from build123d import *

# Parameters (mm, degrees)
SKETCH1_W           = 11
SKETCH1_H           = 12
BOSS_EXTRUDE1_DEPTH = 6.6
CUT_EXTRUDE1_DEPTH  = 6.6


with BuildPart() as part:
    # Sketch1 → Boss-Extrude1 (new body)
    with BuildSketch(Plane(origin=(0, 0, 0), x_dir=(1, 0, 0), z_dir=(0, 1, 0))):
        with Locations((5.5, -6)):
            Rectangle(SKETCH1_W, SKETCH1_H)
    extrude(amount=BOSS_EXTRUDE1_DEPTH)

    # Sketch2 → Cut-Extrude1 (cut)
    with BuildSketch(Plane(origin=(0, 6.6, 0), x_dir=(1, 0, 0), z_dir=(0, 1, 0))):
        with BuildLine():
            ThreePointArc((11, -0.013348181), (9.4, -6), (11, -11.986651819))
            Line((11, -11.986651819), (11, -0.013348181))
        make_face()
        with BuildLine():
            ThreePointArc((0, -11.986651819), (1.6, -6), (0, -0.013348181))
            Line((0, -0.013348181), (0, -11.986651819))
        make_face()
        with BuildLine():
            ThreePointArc((7.275, -6), (6.755114537, -4.744885463), (5.5, -4.225))
            Line((5.5, -4.225), (5.5, -7.775))
            ThreePointArc((5.5, -7.775), (6.755114537, -7.255114537), (7.275, -6))
        make_face()
        with BuildLine():
            Line((5.5, -7.775), (5.5, -4.225))
            ThreePointArc((5.5, -4.225), (3.725, -6), (5.5, -7.775))
        make_face()
    extrude(amount=-CUT_EXTRUDE1_DEPTH, mode=Mode.SUBTRACT)


solid = part.part
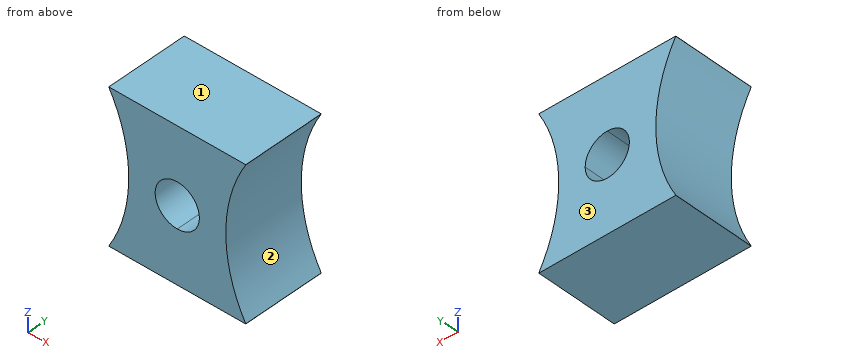
For this review, take the finished solid that the model builds, in its own axes (mm). Face numbers are marked on the shaded views. Round coordinates to 2 decimals unless told otherwise and drop trailing zeros. Loops run counter-clockwise (first coordinate to the right, second up) from the corner with the lowest first, then second, coordinate; pieces in that order, holes last. Notation, with made-up numbers: (40.5, 58) - (48.5, 58) arc R23 ccw to (48.5, 89) - close; hole circle Ø11 at (17, -17.75). An arc over 180 degrees is marked (long way). Put each result on its own line as item: value. Start each with the question number.
1. For probe 1 along Z at (x, y) = (4.5, 2); probe 2 along X at (y, z) = (2.75, 5.25); probe 3 along Z at (x, y) = (6.25, 0.5), list the stretches that pass through material, from the lowest coordinate up. Write a range as [from, to].
2. Consider section A-A on y = 3.75. State the section outline as (x, z) points (3 decimals).
3. Mouldability with a two-part tool opening along Z and no side actions: class the marked faces 1, 2 and 3 as +Z half, -Z half, draft (parallel to the pull), parting line (faces both ways), or undercut.
4. Insertion check: P1, Ø1.5, axis at x = 5.5, z = 6.5, coming from the +Y side; P2, Ø2, axis at y = 3, z = 2, coming from the +X side. Each pin has a flat end and moves straight along its axis. Give the tip position at first contact, or say it passes through.
5. Consider section D-D on z = 9.5. State the section outline as (x, y) points, plus the area to 3 significant figures.
6. Consider section C-C on x = 9.75. State the section outline as (y, z) points.
7. Consider section B-B on z = 7. State the section outline as (x, y) points.
Result sheet:
1. probe 1: [0, 4.53], [7.47, 12]
1. probe 2: [1.58, 3.89], [7.11, 9.42]
1. probe 3: [0, 4.39], [7.61, 12]
2. outline: (0, 0) - (11, 0) - (11, 0.013) arc R12 cw to (11, 11.987) - (11, 12) - (0, 12) - (0, 11.987) arc R12 cw to (0, 0.013) - close; hole circle Ø3.55 at (5.5, 6)
3. face 1: +Z half
3. face 2: undercut
3. face 3: draft
4. P1: through
4. P2: x = 10.49
5. outline: (1.08, 0) - (9.92, 0) - (9.92, 6.6) - (1.08, 6.6) - close
5. area: 58.4 mm^2
6. outline: (0, 0) - (6.6, 0) - (6.6, 3.12) - (0, 3.12) - close; (0, 8.88) - (6.6, 8.88) - (6.6, 12) - (0, 12) - close
7. outline: (1.56, 0) - (4.03, 0) - (4.03, 6.6) - (1.56, 6.6) - close; (6.97, 0) - (9.44, 0) - (9.44, 6.6) - (6.97, 6.6) - close
